Verification items for the finished model (mm, model axes). A direction names the side the tool comes from. Coordinates: 2 decimals unless noted, no trailing zeros. Order: outer loops, then holes, each group sorted by start corner. A loop starts at its lowest first (then second) coordinate and runs counter-clockwise, first axis right, second up. Notation, with made-up numbers: M 46,-27.5 L 99,-27.5 A20 cw 99,5.5 Z; hole C 62.25,39.5 d9. An arc over 180 degrees is marked long. Answer as a JSON object with one key per item and string values. Group by question number.
(1) Cross-section at A-A (y = 8.5). Enter the section's corners in (x, z).
(2) Cross-section at B-B (z = 0). Enter the section's corners in (x, y), plus the area to 3 significant figures.
(3) Mould release check, pull along X, two halves, no side actions. Record for faces 1 (the face through (14.5, 6, 0)), 2 (the face through (7, 8, 0)), 3 (the face through (9, 5, 0)), 4 (the face through (4.5, 6, 0)): released by +X, released by -X, zero draft, split by the parting line, or undercut.
(4) Access from +Z, -Z, +X, -X, +Y, -Y to the whole of each face (thin tool, end or side, straight path). Record for faces 5 (the face through (19, 0, 0)), 6 (the face through (9.367, -2.395, -1.246)).
(5) Cross-section at C-C (x = 10.5). Enter the section's corners in (y, z), plus the area to 3 significant figures.
(6) Material ranges on line 1 (Z direction, x = 9.5, y = 6.9); line 2 (X direction, y = 7.6, z = 0); line 3 (Z direction, x = 9, y = 7), recorded low to high.
(7) Cross-section at D-D (y = 2.5). Enter the section's corners in (x, z).
(8) Gauge pin test, flat ends, axial feed: pin 1 Ø2 at (y, z) = (5.5, 1.5) entering from +X; pin 2 Ø2.5 at (x, z) = (9.5, 0) entering from +Y; pin 3 Ø2 at (y, z) = (4.5, -2) entering from -X. Record the tip position at first contact, or that the pin passes through.
from build123d import *

# Parameters (mm, degrees)
SKETCH1_R           = 2.7
BOSS_EXTRUDE1_DEPTH = 19
SKETCH2_W           = 10
SKETCH2_H           = 5.4
BOSS_EXTRUDE2_DEPTH = 10
SKETCH3_R           = 2.5
CUT_EXTRUDE1_DEPTH  = 5


with BuildPart() as part:
    # Sketch1 → Boss-Extrude1 (new body)
    with BuildSketch(Plane(origin=(0, 0, 0), x_dir=(0, 0, -1), z_dir=(1, 0, 0))):
        Circle(SKETCH1_R)
    extrude(amount=BOSS_EXTRUDE1_DEPTH)

    # Sketch2 → Boss-Extrude2 (add)
    with BuildSketch(Plane(origin=(0, 0, 0), x_dir=(1, 0, 0), z_dir=(0, 1, 0))):
        with Locations((9.5, 0)):
            Rectangle(SKETCH2_W, SKETCH2_H)
    extrude(amount=BOSS_EXTRUDE2_DEPTH)

    # Sketch3 → Cut-Extrude1 (cut)
    with BuildSketch(Plane(origin=(0, 10, 0), x_dir=(1, 0, 0), z_dir=(0, 1, 0))):
        with Locations((9.5, 0)):
            Circle(SKETCH3_R)
    extrude(amount=-CUT_EXTRUDE1_DEPTH, mode=Mode.SUBTRACT)


solid = part.part
Taken from the geometry:
{
 "1": {"outline": "M 4.5,-2.7 L 14.5,-2.7 L 14.5,2.7 L 4.5,2.7 Z; hole C 9.5,0 d5"},
 "2": {"outline": "M 0,-2.7 L 19,-2.7 L 19,2.7 L 14.5,2.7 L 14.5,10 L 12,10 L 12,5 L 7,5 L 7,10 L 4.5,10 L 4.5,2.7 L 0,2.7 Z", "area": "151 mm²"},
 "3": {"face 1": "released by +X", "face 2": "undercut", "face 3": "undercut", "face 4": "released by -X"},
 "4": {"face 5": "+Z, -Z, +X, +Y, -Y", "face 6": "none"},
 "5": {"outline": "M 0,-2.7 L 10,-2.7 L 10,-2.29 L 5,-2.29 L 5,2.29 L 10,2.29 L 10,2.7 L 0,2.7 A2.7 ccw Z", "area": "42.5 mm²"},
 "6": {"line 1": "z = -2.7 to -2.5, 2.5 to 2.7", "line 2": "x = 4.5 to 7, 12 to 14.5", "line 3": "z = -2.7 to -2.45, 2.45 to 2.7"},
 "7": {"outline": "M 0,-1.02 L 4.5,-1.02 L 4.5,-2.7 L 14.5,-2.7 L 14.5,-1.02 L 19,-1.02 L 19,1.02 L 14.5,1.02 L 14.5,2.7 L 4.5,2.7 L 4.5,1.02 L 0,1.02 Z"},
 "8": {"pin 1": "stops at x = 14.5", "pin 2": "stops at y = 5", "pin 3": "stops at x = 4.5"}
}
